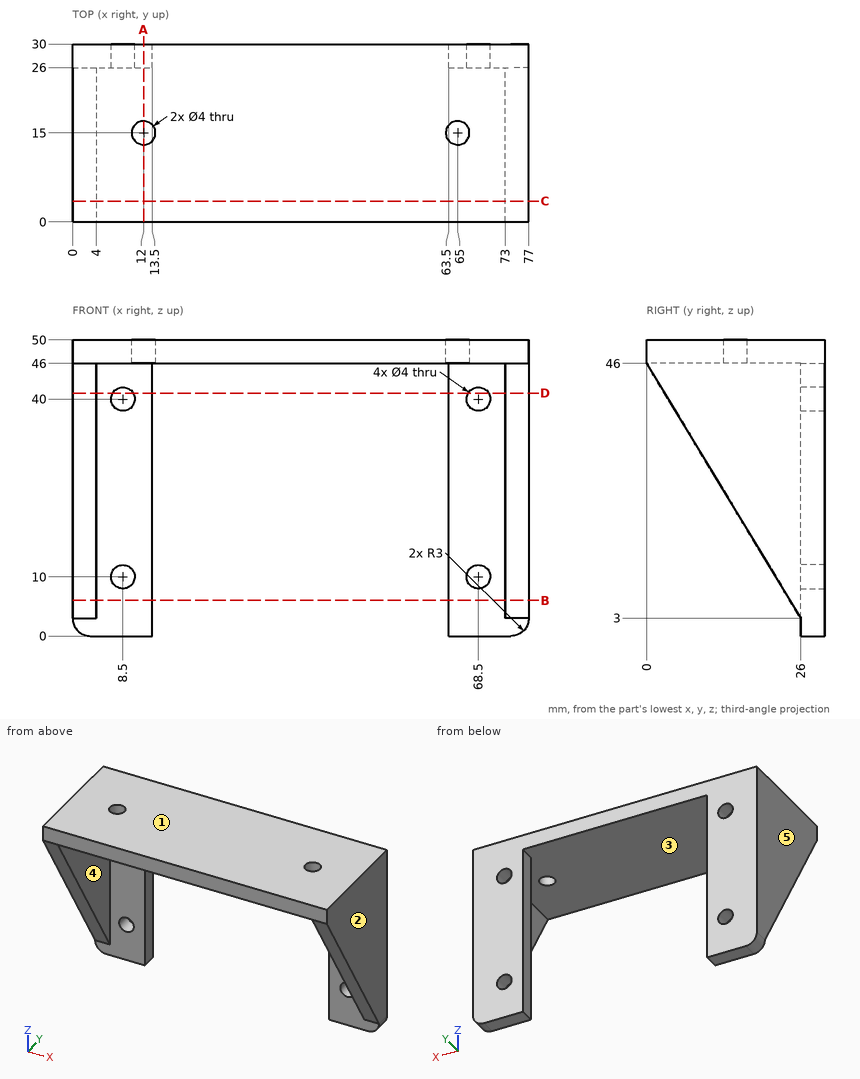
Answer from the drawing. Dimensions are ordinates in mm from the lowest x, y and z of the part. A direction names the side the tool comes from. Round coordinates to 2 decimals unless told otherwise and drop trailing zeros. Loops run counter-clockwise (first coordinate to the right, second up) from the corner with the lowest first, then second, coordinate; pieces in that order, holes last.
Q1. Section B-B on z = 6 is taken. Write down the section's boundary in (x, y).
Q2. Which of the six approach directions +Z, -Z, +X, -X, +Y, -Y give full straight-line access (tool end or side, diameter ignored) to the marked faces 4 and 5?
Q3. Section A-A on x = 12 is taken. Write down the section's boundary in (y, z), and give its area (3 significant figures).
Q4. Each of these flat-tipped pins is pushed along its axis until it touches: pin 1 (7 mm diameter, centred on x = 73.5, z = 12, fed in from -Y); pin 2 (10 mm diameter, centred on x = 65, y = 24, fed in from -Z); pin 3 (3 mm diameter, centred on x = 36, y = 26.5, fed in from -Z). Where does it stop, or does it pass through?
Q5. Section D-D on z = 41 is taken. Write down the section's boundary in (x, y).
Q6. Section C-C on y = 3.5 is taken. Write down the section's boundary in (x, z).
Q7. Determine the mould class of the marked faces 1, 2 and 3 for opening direction X: released by +X, released by -X, zero draft, split by the parting line, or undercut.
Q8. Consider probe 1 along Z at (x, y) = (68.5, 28.7); probe 2 along X at (y, z) = (29.1, 10); probe 3 along X at (y, z) = (20.25, 38). Determine where each line is inside the solid, lowest interval first.
Output:
1. outline: (0, 24.19) - (4, 24.19) - (4, 26) - (13.5, 26) - (13.5, 30) - (0, 30) - close; (63.5, 26) - (73, 26) - (73, 24.19) - (77, 24.19) - (77, 30) - (63.5, 30) - close
2. face 4: -Z, -Y
2. face 5: +Z, -Z, -X, +Y, -Y
3. outline: (0, 46) - (13, 46) - (13, 50) - (0, 50) - close; (17, 46) - (26, 46) - (26, 0) - (30, 0) - (30, 50) - (17, 50) - close
3. area: 288 mm2
4. pin 1: stops at y = 18.44
4. pin 2: stops at z = 0
4. pin 3: stops at z = 46
5. outline: (0, 3.02) - (4, 3.02) - (4, 26) - (6.77, 26) - (6.77, 30) - (0, 30) - close; (10.23, 26) - (13.5, 26) - (13.5, 30) - (10.23, 30) - close; (63.5, 26) - (66.77, 26) - (66.77, 30) - (63.5, 30) - close; (70.23, 26) - (73, 26) - (73, 3.02) - (77, 3.02) - (77, 30) - (70.23, 30) - close
6. outline: (0, 40.21) - (4, 40.21) - (4, 46) - (73, 46) - (73, 40.21) - (77, 40.21) - (77, 50) - (0, 50) - close
7. face 1: zero draft
7. face 2: released by +X
7. face 3: undercut
8. probe 1: z = 0 to 8, 12 to 38, 42 to 50
8. probe 2: x = 0 to 6.5, 10.5 to 13.5, 63.5 to 66.5, 70.5 to 77
8. probe 3: x = 0 to 4, 73 to 77
